Verification items for the finished model (mm, model axes). Face numbers are marked on the shaded views. A direction names the side the tool comes from. Give positions to 0.01 mm unless a question says otherwise; leave off trailing zeros. Order: outer loops, then holes, each group sorted by start corner. A loop starts at its lowest first (then second) coordinate and runs counter-clockwise, first axis right, second up.
(1) Scan lines: L1, parallel to X at y = 0, z = 5; L2, parallel to Y at x = 0, z = 1.2 (3 decimals). Record each from-to range of solid material in increasing order.
(2) Sectioned sample at C-C on y = 6.5. Record the cut outline in (x, z), plus the area to 3 significant figures.
(3) Access from +Z, -Z, +X, -X, +Y, -Y to the whole of each face (thin tool, end or side, straight path). Record for the marked faces 1 and 2.
(4) Sectioned sample at D-D on z = 3.5. Record the cut outline in (x, y), plus the area to 3 significant figures.
(5) Sectioned sample at B-B on z = 24.5. Record the cut outline in (x, y).
(6) Gauge pin test, flat ends, axial feed: pin 1 (4.5 mm diameter, centred on x = 2, y = 1.5, fed in from +Z); pin 2 (3 mm diameter, centred on x = -10.5, z = 17.5, fed in from -Y); pin 3 (12 mm diameter, centred on x = 7.5, z = 12, fed in from -Y). Record the tip position at first contact, or that the pin passes through.
(7) Sectioned sample at A-A on y = 2.25. Record the cut outline in (x, z).
```python
from build123d import *
from build123d.topology import SkipClean

# Parameters (mm, degrees)
SKETCH1_R           = 7.5
SKETCH1_R_2         = 3.285
BOSS_EXTRUDE1_DEPTH = 2
SKETCH1_3_R         = 10
SKETCH1_3_R_2       = 7.5
BOSS_EXTRUDE2_DEPTH = 14
BOSS_EXTRUDE3_DEPTH = 10
BOSS_EXTRUDE4_DEPTH = 10
SKETCH4_R           = 1.8
CUT_EXTRUDE1_DEPTH  = 10
FILLET1_R           = 2
FILLET2_R           = 2


with BuildPart() as part:
    # Sketch1 → Boss-Extrude1 (new body)
    with BuildSketch(Plane.XY):
        Circle(SKETCH1_R)
        Circle(SKETCH1_R_2, mode=Mode.SUBTRACT)
    extrude(amount=BOSS_EXTRUDE1_DEPTH)

    # Sketch1<3> → Boss-Extrude2 (add)
    with BuildSketch(Plane.XY):
        Circle(SKETCH1_3_R)
        Circle(SKETCH1_3_R_2, mode=Mode.SUBTRACT)
    extrude(amount=BOSS_EXTRUDE2_DEPTH)

    # Sketch2 → Boss-Extrude3 (add)
    with SkipClean():  # the faces are left unmerged after this step: merging them gives an invalid solid
        with BuildSketch(Plane.XY.offset(14)):
            with BuildLine():
                ThreePointArc((0.880723614, 9.961140794), (-9.097879067, 4.150734451), (-6.945976325, -7.193984493))
                Line((-6.945976325, -7.193984493), (-5.209482244, -5.39548837))
                ThreePointArc((-5.209482244, -5.39548837), (-6.8234093, 3.113050838), (0.66054271, 7.470855595))
                Line((0.66054271, 7.470855595), (0.880723614, 9.961140794))
            make_face()
            with BuildLine():
                Line((-0.66054271, -7.470855595), (-0.880723614, -9.961140794))
                ThreePointArc((-0.880723614, -9.961140794), (6.752509306, -7.375880833), (10, 0))
                ThreePointArc((10, 0), (9.204883575, 3.907699883), (6.945976325, 7.193984493))
                Line((6.945976325, 7.193984493), (5.209482244, 5.39548837))
                ThreePointArc((5.209482244, 5.39548837), (6.903662681, 2.930774912), (7.5, 0))
                ThreePointArc((7.5, 0), (5.06438198, -5.531910625), (-0.66054271, -7.470855595))
            make_face()
        extrude(amount=BOSS_EXTRUDE3_DEPTH)

    # Sketch3 → Boss-Extrude4 (add)
    with SkipClean():  # the faces are left unmerged after this step: merging them gives an invalid solid
        with BuildSketch(Plane.XY.offset(24)):
            Polygon((8.437336357, -11.621590046), (7.458998865, -13.765980707), (-15.285698803, -3.38914458), (-14.307361311, -1.244753919), align=None)
        extrude(amount=BOSS_EXTRUDE4_DEPTH)

    # Sketch4 → Cut-Extrude1 (cut)
    with SkipClean():  # the faces are left unmerged after this step: merging them gives an invalid solid
        with BuildSketch(Plane(origin=(-3.913349969, -8.577562644, 0), x_dir=(0.9097879067131455, -0.4150734450654641, 0), z_dir=(-0.4150734450654641, -0.9097879067131455, 0))):
            with Locations((-5, 29)):
                Circle(SKETCH4_R)
            with Locations((5, 29)):
                Circle(SKETCH4_R)
        extrude(amount=-CUT_EXTRUDE1_DEPTH, mode=Mode.SUBTRACT)

    # Fillet1
    # the kernel refuses this fillet: 2 mm, written as the material it adds along each edge
    with BuildSketch(Plane(origin=(-5.209482244, -5.39548837, 24), x_dir=(0.415073445065464, 0.9097879067131456, 0), z_dir=(0.9097879067131456, -0.415073445065464, 0))) as fillet1_piece_1_section:
        with BuildLine():
            CenterArc((FILLET1_R, FILLET1_R), FILLET1_R, 180, 90)
            Line((0, FILLET1_R), (0, 0))
            Line((0, 0), (FILLET1_R, 0))
        make_face()
    fillet1_piece_1 = extrude(amount=14.571067812, mode=Mode.PRIVATE)
    fillet1_piece_1 = fillet1_piece_1 & Plane(origin=(0, 0, 24.466684855), x_dir=(-0.08807236135728662, -0.9961140793929938, 0), z_dir=(0, 0, -1)) * Cylinder(10, 38, mode=Mode.PRIVATE)
    fillet1_piece_1 = fillet1_piece_1 - Plane(origin=(0, 0, 24.466684855), x_dir=(0.6945976324993828, 0.7193984493493522, 0), z_dir=(0, 0, -1)) * Cylinder(7.5, 38, mode=Mode.PRIVATE)
    add(fillet1_piece_1)
    with BuildSketch(Plane(origin=(-13.917123993, -1.42279228, 24), x_dir=(0.415073445065464, 0.9097879067131456, 0), z_dir=(0.9097879067131456, -0.415073445065464, 0))) as fillet1_piece_2_section:
        with BuildLine():
            CenterArc((FILLET1_R, FILLET1_R), FILLET1_R, 180, 90)
            Line((0, FILLET1_R), (0, 0))
            Line((0, 0), (FILLET1_R, 0))
        make_face()
    fillet1_piece_2 = extrude(amount=14.571067812, mode=Mode.PRIVATE)
    fillet1_piece_2 = fillet1_piece_2 & Plane(origin=(0, 0, 24.466680249), x_dir=(0.08807236135728662, 0.9961140793929938, 0), z_dir=(0, 0, -1)) * Cylinder(10, 38, mode=Mode.PRIVATE)
    fillet1_piece_2 = fillet1_piece_2 - Plane(origin=(0, 0, 24.466680249), x_dir=(0.6945976324993828, 0.7193984493493522, 0), z_dir=(0, 0, -1)) * Cylinder(7.5, 38, mode=Mode.PRIVATE)
    add(fillet1_piece_2)

    # Fillet2
    # the kernel refuses this fillet: 2 mm, written as the material it adds along each edge
    with BuildSketch(Plane(origin=(0, 0, 24), x_dir=(0.7561376391606037, -0.6544126149797455, 0), z_dir=(0.6544126149797455, 0.7561376391606037, 0))) as fillet2_piece_1_section:
        with BuildLine():
            CenterArc((10 + FILLET2_R, FILLET2_R), FILLET2_R, 180, 90)
            Line((10 + FILLET2_R, 0), (10, 0))
            Line((10, 0), (10, FILLET2_R))
        make_face()
    fillet2_piece_1 = revolve(axis=Axis((0, 0, 24), (0, 0, -1)), revolution_arc=82.826410261, mode=Mode.PRIVATE)
    fillet2_piece_1 = split(fillet2_piece_1, bisect_by=Plane(origin=(2.607194883, -8.96169878, 23.537511389), z_dir=(-0.415073445065464, -0.9097879067131456, 0)), keep=Keep.TOP, mode=Mode.PRIVATE)
    fillet2_piece_1 = split(fillet2_piece_1, bisect_by=Plane(origin=(1.628857391, -11.106089441, 23.537511389), z_dir=(0.41507344506546406, 0.9097879067131456, 0)), keep=Keep.TOP, mode=Mode.PRIVATE)
    add(fillet2_piece_1)
    with BuildSketch(Plane(origin=(0, 0, 24), x_dir=(-0.9898439357335846, 0.1421583022248339, 0), z_dir=(0.1421583022248339, 0.9898439357335846, 0))) as fillet2_piece_2_section:
        with BuildLine():
            CenterArc((10 + FILLET2_R, -FILLET2_R), FILLET2_R, 90, 90)
            Line((10 + FILLET2_R, 0), (10, 0))
            Line((10, 0), (10, -FILLET2_R))
        make_face()
    fillet2_piece_2 = revolve(axis=Axis((0, 0, 24), (0, 0, 1)), revolution_arc=82.826410261, mode=Mode.PRIVATE)
    fillet2_piece_2 = split(fillet2_piece_2, bisect_by=Plane(origin=(-8.477218422, -3.904645831, 23.537511225), z_dir=(-0.415073445065464, -0.9097879067131456, 0)), keep=Keep.TOP, mode=Mode.PRIVATE)
    fillet2_piece_2 = split(fillet2_piece_2, bisect_by=Plane(origin=(-9.455555915, -6.049036492, 23.537511225), z_dir=(0.41507344506546406, 0.9097879067131456, 0)), keep=Keep.TOP, mode=Mode.PRIVATE)
    add(fillet2_piece_2)


solid = part.part
```
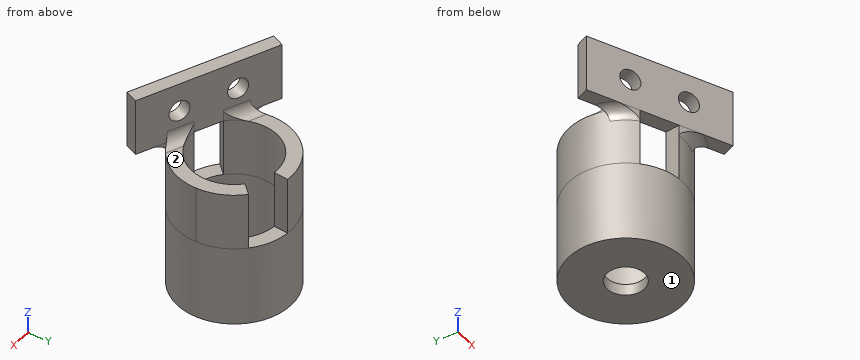
Ans:
1. L1: x = -10 to -7.5, 7.5 to 10
1. L2: y = -10 to -3.285, 3.285 to 10
2. outline: (-7.6, 0) - (7.6, 0) - (7.6, 24) - (6.28, 24) - (6.28, 14) - (3.74, 14) - (3.74, 2) - (-3.74, 2) - (-3.74, 24) - (-7.6, 24) - close
2. area: 175 mm2
3. face 1: -Z, +X, -X, +Y, -Y
3. face 2: +Z, +X, +Y
4. outline: circle Ø20 at (0, 0); hole circle Ø15 at (0, 0)
4. area: 137 mm2
5. outline: (-15.29, -3.39) - (7.46, -13.77) - (8.44, -11.62) - (3.5, -9.37) arc R10 ccw to (4.34, -9.01) - (0.91, -7.44) arc R7.5 cw to (-0.66, -7.47) - (-5.21, -5.4) arc R7.5 cw to (-6.22, -4.19) - (-9.65, -2.63) arc R10 ccw to (-9.37, -3.5) - (-14.31, -1.24) - close
6. pin 1: stops at z = 2
6. pin 2: stops at y = -4.36
6. pin 3: stops at y = -9.89
7. outline: (-9.74, 0) - (-2.39, 0) - (-2.39, 2) - (-7.15, 2) - (-7.15, 24) - (-9.74, 24) - close; (2.39, 0) - (9.74, 0) - (9.74, 24) - (7.15, 24) - (7.15, 2) - (2.39, 2) - close
